Part model, mm, in its own coordinate system. A direction names the side the tool comes from. Coordinates: 2 decimals unless noted, no trailing zeros. Write each loop counter-clockwise with the first axis right and the second up, starting at its lowest first coordinate (ties: lowest second). Pieces come first, ordered by that corner, then holes. Notation, with made-up numbers: M 76.25,49.25 L 128.25,49.25 A15 cw 128.25,59.25 Z; hole C 43,-19 d10. An arc over 180 degrees is marked long. Use a Markdown table: item, result. Add a question column.
Q1. Slice it at A-A on y = -40. Write the cut outline in (x, z).
Q2. Slice it at B-B on x = 0. Write the cut outline in (y, z), then the cut area to 3 significant figures.
Q3. Pin check, flat tips, straight feed: pin 1 Ø3 at (x, z) = (-11.5, 29) entering from -Y; pin 2 Ø1 at (x, y) = (-20, -17.5) entering from +Z; pin 3 Ø12 at (x, z) = (9, 59.5) entering from -Y. Stop position of each tip, or through.
Q4. Slice it at C-C on y = 0. Write the cut outline in (x, z).
Q5. Tool access for faces 4 (the flat face through (0, 0, 80)), 5 (the flat face through (-15, -11, 15)): list every direction of +Z, -Z, +X, -X, +Y, -Y with a clear straight run to the whole face (end or side of a thin tool).
Q6. Mould opens along Y. For faces 1 (the cylindrical face through (-18.801, -45.857, 7.605)), 2 (the cylindrical face through (-14.985, 0.66, 47.927)), 3 (the flat face through (-32.5, -1, 7)) say: released by +Y, released by -Y, zero draft, split by the parting line, or undercut.
Q7. Wall check: L1, parallel to Y at x = -17.5, z = 7.5; L2, parallel to Z at x = -8, y = -49; L3, parallel to Y at x = 0, z = 49.5. Give the ranges that are in metal, low to high. Write a range as from..to.
Q8. Slice it at D-D on z = 28. Write the cut outline in (x, y).
from build123d import *

# Parameters (mm, degrees)
F0_W      = 65
F0_H      = 110
F1_DEPTH  = 100
F2_W      = 65
F2_H      = 110
F2_R      = 15
F3_DEPTH  = 85
F1_FACE_R = 15
F4_DEPTH  = 20
F5_R      = 6
F6_DEPTH  = 30
F7_R      = 2


with BuildPart() as f1:
    # F0 (on Top) → F1 (new body)
    with BuildSketch(Plane.XY):
        Rectangle(F0_W, F0_H)
    extrude(amount=F1_DEPTH)

    # F2 (on face) → F3 (cut)
    with BuildSketch(Plane.XY.offset(100)):
        Rectangle(F2_W, F2_H)
        Circle(F2_R, mode=Mode.SUBTRACT)
    extrude(amount=-F3_DEPTH, mode=Mode.SUBTRACT)

    # F1_face (on face) → F4 (cut)
    with BuildSketch(Plane.XY.offset(100)):
        Circle(F1_FACE_R)
    extrude(amount=-F4_DEPTH, mode=Mode.SUBTRACT)

    # F5 (on face) → F6 (cut)
    with BuildSketch(Plane.XY.offset(15)):
        with Locations((-17.5, 40)):
            Circle(F5_R)
        with Locations((17.500002, 40)):
            Circle(F5_R)
        with Locations((17.500002, -40)):
            Circle(F5_R)
        with Locations((-17.5, -40)):
            Circle(F5_R)
    extrude(amount=-F6_DEPTH, mode=Mode.SUBTRACT)

    # F7
    f7_edges = [f1.edges().sort_by_distance(p)[0] for p in [
        (-15, 0, 80),
        (-15, 0, 15),
    ]]
    fillet(f7_edges, radius=F7_R)


solid = f1.part
Recorded:
| question | item | result |
|---|---|---|
| 1 | outline | M -32.5,0 L -23.5,0 L -23.5,15 L -32.5,15 Z; M -11.5,0 L 11.5,0 L 11.5,15 L -11.5,15 Z; M 23.5,0 L 32.5,0 L 32.5,15 L 23.5,15 Z |
| 2 | outline | M -55,0 L 55,0 L 55,15 L 17,15 A2 cw 15,17 L 15,78 A2 ccw 13,80 L -13,80 A2 ccw -15,78 L -15,17 A2 cw -17,15 L -55,15 Z |
| 2 | area | 3,600 mm² |
| 3 | pin 1 | y = -11.18 |
| 3 | pin 2 | z = 15 |
| 3 | pin 3 | y = -14.7 |
| 4 | outline | M -32.5,0 L 32.5,0 L 32.5,15 L 17,15 A2 cw 15,17 L 15,78 A2 ccw 13,80 L -13,80 A2 ccw -15,78 L -15,17 A2 cw -17,15 L -32.5,15 Z |
| 5 | face 4 | +Z, +X, -X, +Y, -Y |
| 5 | face 5 | +Z |
| 6 | face 1 | undercut |
| 6 | face 2 | split by the parting line |
| 6 | face 3 | zero draft |
| 7 | L1 | -55..-46, -34..34, 46..55 |
| 7 | L2 | 0..15 |
| 7 | L3 | -15..15 |
| 8 | outline | C 0,0 d30 |
